Print and shaded views of the part. All mm, measured from the part's lowest x, y and z. A direction names the side the tool comes from. Give positions to 0.01 mm unless a question says otherwise; leave off trailing zeros. Loops run counter-clockwise (first coordinate to the right, second up) from the corner with the lowest first, then second, coordinate; pieces in that order, holes last. Notation, with made-up numbers: (-39, 55) - (-24, 55) arc R29 ccw to (-24, 88) - close; hole circle Ø9 at (0, 58). An arc over 180 degrees is marked (long way). Return JSON: item names as keys, results as strings.
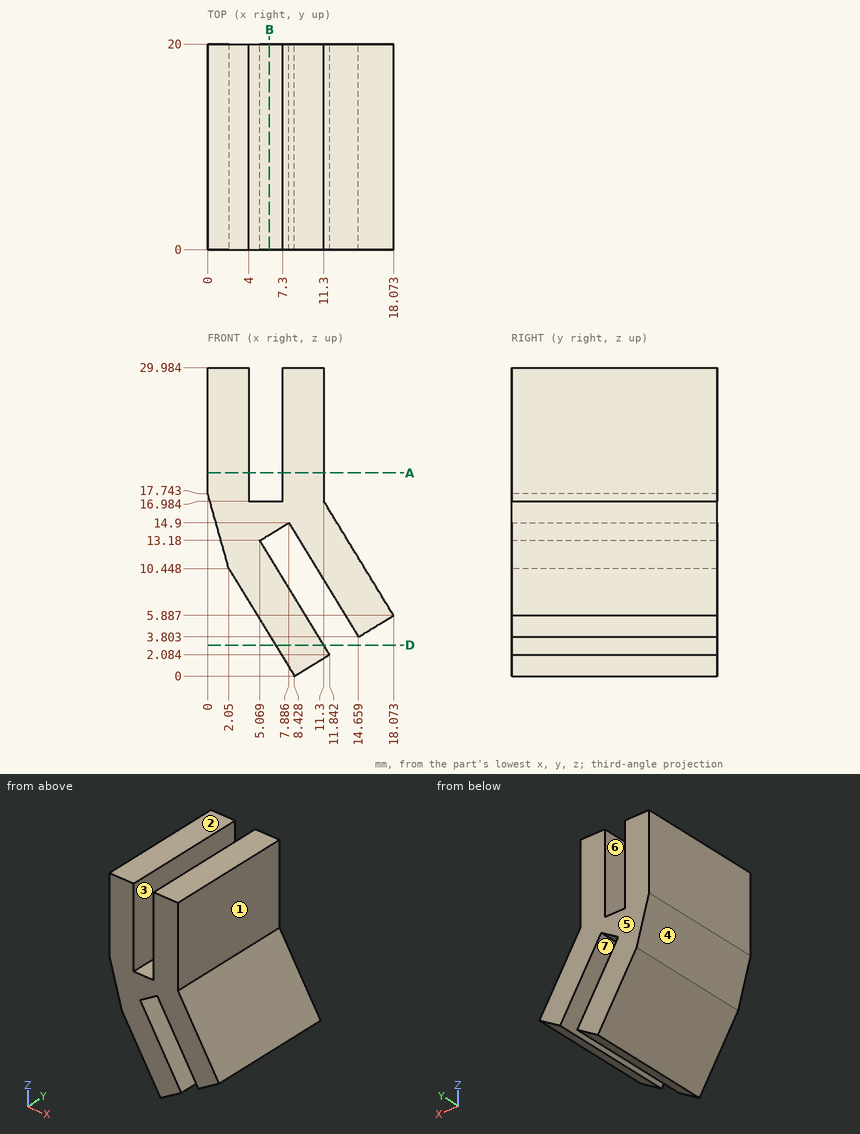
1. Drill centre lines: probe 1 along X at (y, z) = (18.75, 25.75); probe 2 along Z at (x, y) = (11, 15.75) (1 decimal); probe 3 along Z at (x, y) = (10.5, 9.75) (1 decimal). Where is each one in solid material? Low to high.
Values follow:
{"probe 1": "x = 0 to 4, 7.3 to 11.3", "probe 2": "z = 1.6 to 3.5, 9.8 to 30", "probe 3": "z = 1.3 to 4.3, 10.6 to 30"}
2. Cut at A-A, the plane z = 19.75. Write the cut outline in (x, y).
Values follow:
{"outline": "(0, 0) - (4, 0) - (4, 20) - (0, 20) - close; (7.3, 0) - (11.3, 0) - (11.3, 20) - (7.3, 20) - close"}
3. Which spindle directions (+Z, -Z, +X, -X, +Y, -Y) get a long thin tool onto all of the face, cutting with end or side? Do the marked faces 5, 6 and 7. Say none if no direction does.
Values follow:
{"face 5": "+Z, -Z, +X, -X, +Y", "face 6": "+Z, +Y, -Y", "face 7": "+Y, -Y"}
4. Pull direction X, two halves, no side cores. Call the marked faces 1, 2, 3 and 4: +X half, -X half, draft (parallel to the pull), parting line (faces both ways), or undercut.
Values follow:
{"face 1": "+X half", "face 2": "draft", "face 3": "undercut", "face 4": "-X half"}
5. Cut at D-D, the plane z = 3. Write the cut outline in (x, y).
Values follow:
{"outline": "(6.6, 0) - (11.28, 0) - (11.28, 20) - (6.6, 20) - close"}
6. Cut at B-B, the plane x = 6. Write the cut outline in (y, z) (1 decimal), plus the area to 3 significant figures.
Values follow:
{"outline": "(0, 4) - (20, 4) - (20, 11.7) - (0, 11.7) - close; (0, 13.7) - (20, 13.7) - (20, 17) - (0, 17) - close", "area": "218 mm²"}
7. Drop flat-ended pins along their axis: P1, Ø1, axis at x = 6, y = 5.5, coming from the +Z side; P2, Ø1, axis at y = 8, z = 26, coming from the +X side; P3, Ø5, axis at x = 14.5, y = 11, coming from the +Z side (1 decimal). Give the stop position or say it passes through.
Values follow:
{"P1": "stops at z = 16.98", "P2": "stops at x = 11.3", "P3": "stops at z = 15.8"}
